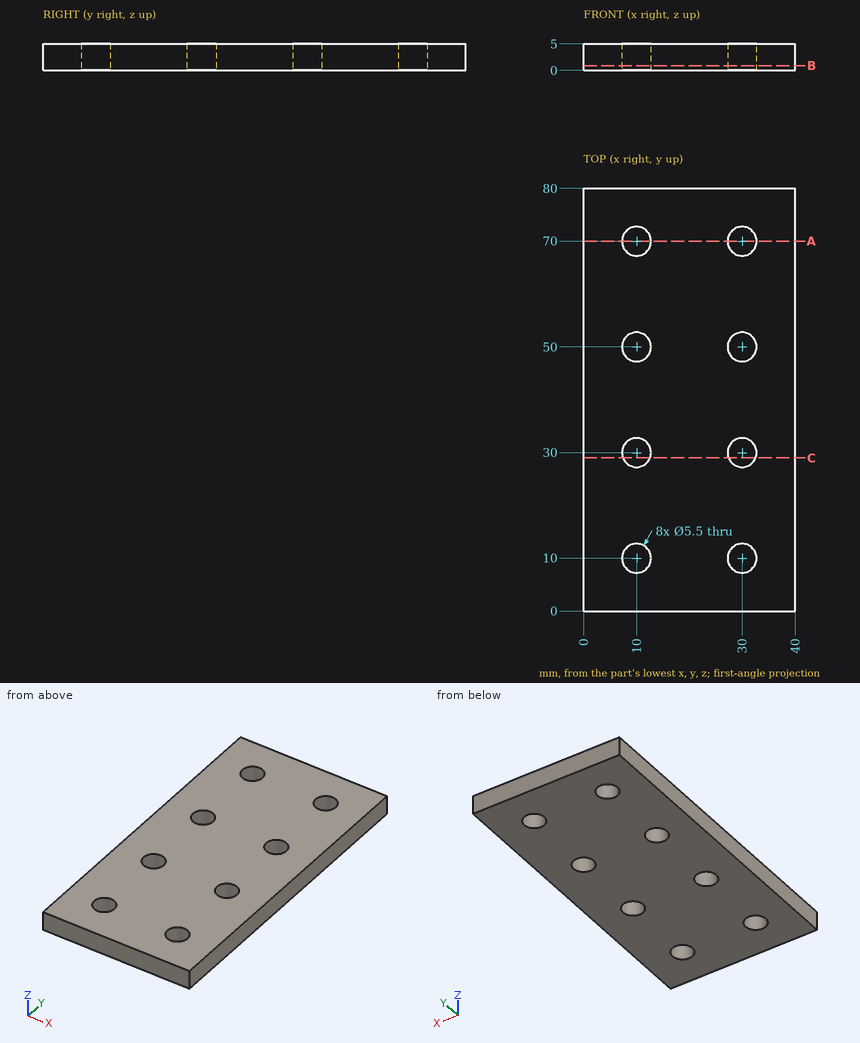
Design review of the part shown in the three views and the two pictorial views. Dimensions are in mm from the part's minimum x, y and z. Give positions to 0.01 mm unless a question says otherwise; leave off trailing zeros. Loops run counter-clockwise (first coordinate to the right, second up) from the corner with the lowest first, then second, coordinate; pieces in that order, holes last. Notation, with made-up numbers: M 50.5,7.25 L 63.5,7.25 A22 cw 63.5,24.25 Z; hole C 53,-16.75 d8. An arc over 180 degrees is marked long. Write item = value, one per line.
Q1. We need section A-A (y = 70). Give the boundary of the cut face in (x, z), plus the area to 3 significant figures.
Output values:
outline = M 0,0 L 7.25,0 L 7.25,5 L 0,5 Z; M 12.75,0 L 27.25,0 L 27.25,5 L 12.75,5 Z; M 32.75,0 L 40,0 L 40,5 L 32.75,5 Z
area = 145 mm^2
Q2. We need section C-C (y = 29). Give the boundary of the cut face in (x, z), plus the area to 3 significant figures.
Output values:
outline = M 0,0 L 7.44,0 L 7.44,5 L 0,5 Z; M 12.56,0 L 27.44,0 L 27.44,5 L 12.56,5 Z; M 32.56,0 L 40,0 L 40,5 L 32.56,5 Z
area = 149 mm^2
Q3. We need section B-B (z = 0.9). Count the separate pieces of the cut face and the enclosed holes in it, plus the area to 3 significant figures.
Output values:
separate_pieces = 1
enclosed_holes = 8
area = 3,010 mm^2
Q4. To check wall thickness, follow line 1 (Y direction, x = 30, z = 1.2); line 2 (X direction, y = 49, z = 3); line 3 (X direction, y = 72, z = 3.3). State the ranges of each line that lie inside material, in increasing order. Write a range as [from, to].
Output values:
line_1 = [0, 7.25], [12.75, 27.25], [32.75, 47.25], [52.75, 67.25], [72.75, 80]
line_2 = [0, 7.44], [12.56, 27.44], [32.56, 40]
line_3 = [0, 8.11], [11.89, 28.11], [31.89, 40]
Q5. Insertion check: pin 1 (5 mm diameter, centred on x = 10, y = 50, fed in from -Z). The pin has a flat end and moves straight along its axis. Give the tip position at first contact, or say it passes through.
Output values:
pin_1 = through
